Check sheet for the drawn part. Datum: minimum x, y, z corner. Units: mm. Round coordinates to 2 decimals unless told otherwise and drop trailing zeros. Order: outer loops, then holes, each group sorted by start corner. A loop starts at its lowest first (then second) coordinate and runs counter-clockwise, first axis right, second up. Notation, with made-up numbers: (-37, 35.5) - (-33, 35.5) arc R27 cw to (-33, 60.5) - close; hole circle Ø4 at (-22, -15). An arc over 180 degrees is marked (long way). Write each question's results on one line, items separated by ' | '.
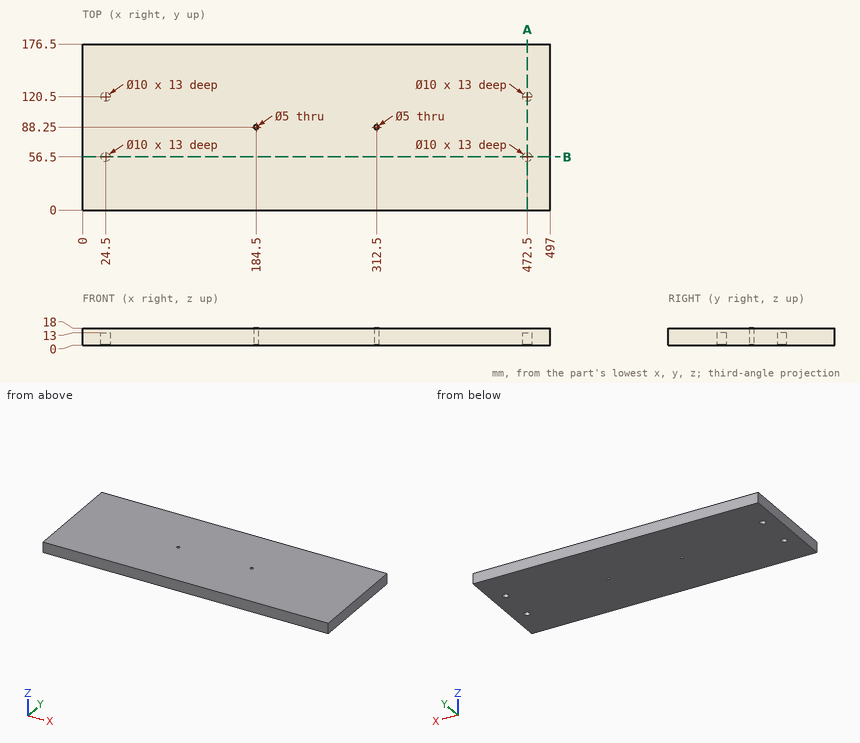
(1) Section check B-B (y = 56.5). Record the cut outline in (x, z).
Answers follow:
outline: (0, 0) - (19.5, 0) - (19.5, 13) - (29.5, 13) - (29.5, 0) - (467.5, 0) - (467.5, 13) - (477.5, 13) - (477.5, 0) - (497, 0) - (497, 18) - (0, 18) - close
(2) Material ranges on line 1 (Y direction, x = 472.5, z = 10.75); line 2 (X direction, y = 120.5, z = 7.25); line 3 (X direction, y = 121.5, z = 10.5), recorded low to high.
Answers follow:
line 1: 0 to 51.5, 61.5 to 115.5, 125.5 to 176.5 | line 2: 0 to 19.5, 29.5 to 467.5, 477.5 to 497 | line 3: 0 to 19.6, 29.4 to 467.6, 477.4 to 497
(3) Depth check by flat-ended pin: pin 1 Ø3 at (x, y) = (474, 118.5) entering from -Z. Enter the tip coordinate at first touch or a pass-through.
Answers follow:
pin 1: z = 13
(4) Section check A-A (x = 472.5). Record the cut outline in (y, z).
Answers follow:
outline: (0, 0) - (51.5, 0) - (51.5, 13) - (61.5, 13) - (61.5, 0) - (115.5, 0) - (115.5, 13) - (125.5, 13) - (125.5, 0) - (176.5, 0) - (176.5, 18) - (0, 18) - close
